Could you check a few things on this model? Use its own coordinates, in mm. Round coordinates to 2 decimals unless told otherwise and drop trailing zeros. Write each loop counter-clockwise with the first axis right and the second up, starting at its lowest first coordinate (ties: lowest second). Pieces come first, ordered by that corner, then holes. Notation, with made-up numbers: (88.5, 77) -> (125.5, 77) arc R5 ccw to (125.5, 85) -> close; hole circle Ø5 at (75.25, 56.25). An arc over 180 degrees is marked (long way). Answer as CSV lines item,"result". Start each with the question number.
Q1. If I drill on line 1 (X direction, y = -1, z = 516); line 2 (Y direction, x = -9.75, z = 141.5); line 3 (Z direction, x = -11.25, y = 10.5), over which ranges is the centre line in solid material (lowest first)? Write a range as [from, to].
Q2. Imagine slicing it at A-A on y = 1.25. Please give me the cut outline in (x, z), and give its area (3 significant figures).
Q3. Imagine slicing it at C-C on z = 499.5. Please give me the cut outline in (x, y), and give its area (3 significant figures).
Q4. Imagine slicing it at B-B on x = -2. Please give me the cut outline in (y, z), and give its area (3 significant figures).
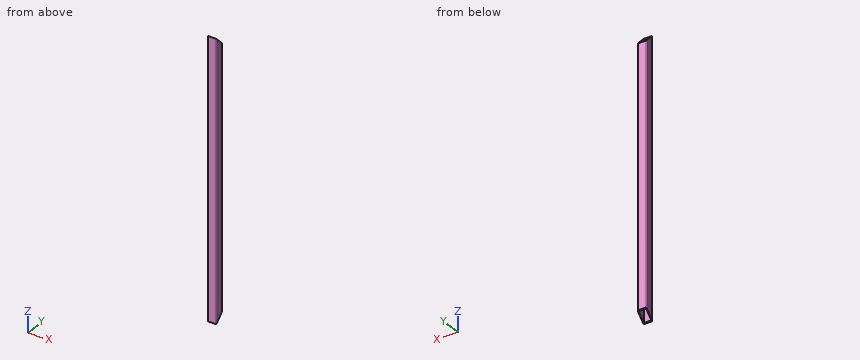
from build123d import *

# Parameters (mm, degrees)
F0_W     = 21
F0_H     = 21
F1_DEPTH = 800
F3_DEPTH = 12.5


with BuildPart() as f1:
    # F0 (on Top) → F1 (new body)
    with BuildSketch(Plane.XY):
        with BuildLine():
            ThreePointArc((12.5, 9.5), (11.62132, 11.62132), (9.5, 12.5))
            Line((9.5, 12.5), (-9.5, 12.5))
            ThreePointArc((-9.5, 12.5), (-11.62132, 11.62132), (-12.5, 9.5))
            Line((-12.5, 9.5), (-12.5, -9.5))
            ThreePointArc((-12.5, -9.5), (-11.62132, -11.62132), (-9.5, -12.5))
            Line((-9.5, -12.5), (9.5, -12.5))
            ThreePointArc((9.5, -12.5), (11.62132, -11.62132), (12.5, -9.5))
            Line((12.5, -9.5), (12.5, 9.5))
        make_face()
        Rectangle(F0_W, F0_H, mode=Mode.SUBTRACT)
    extrude(amount=F1_DEPTH)

    # F2 (on Right) → F3 (cut, symmetric)
    with BuildSketch(Plane.YZ):
        Polygon((12.5, 25), (-12.5, 0), (12.5, 0), align=None)
        Polygon((-12.5, 770.5), (12.5, 745.5), (12.5, 800), (-12.5, 800), align=None)
    extrude(amount=F3_DEPTH, both=True, mode=Mode.SUBTRACT)


solid = f1.part
Checks:
1,line 1,"[-12.5, -10.5], [10.5, 12.5]"
1,line 2,"[-12.49, -10.5], [10.5, 12.49]"
1,line 3,"[23, 747.5]"
2,outline,"(-12.5, 13.75) -> (-10.5, 13.75) -> (-10.5, 756.75) -> (-12.5, 756.75) -> close; (10.5, 13.75) -> (12.5, 13.75) -> (12.5, 756.75) -> (10.5, 756.75) -> close"
2,area,"2,970 mm^2"
3,outline,"(-12.5, -9.5) arc R3 ccw to (-9.5, -12.5) -> (9.5, -12.5) arc R3 ccw to (12.5, -9.5) -> (12.5, 9.5) arc R3 ccw to (9.5, 12.5) -> (-9.5, 12.5) arc R3 ccw to (-12.5, 9.5) -> close; hole (-10.5, -10.5) -> (10.5, -10.5) -> (10.5, 10.5) -> (-10.5, 10.5) -> close"
3,area,"176 mm^2"
4,outline,"(-12.5, 0) -> (-10.5, 2) -> (-10.5, 768.5) -> (-12.5, 770.5) -> close; (10.5, 23) -> (12.5, 25) -> (12.5, 745.5) -> (10.5, 747.5) -> close"
4,area,"2,980 mm^2"
